```python
from build123d import *

# Parameters (mm, degrees)
SKETCH1_W                 = 108.8
SKETCH1_H                 = 23
MOUNT_BASE_DEPTH          = 5
SKETCH2_R                 = 1
SKETCH2_R_2               = 4.5
BRACKET_SCREW_HOLES_DEPTH = 5
SKETCH3_R                 = 1.5875
ANTENNA_SCREW_HOLES_DEPTH = 5


with BuildPart() as part:
    # Sketch1 → Mount Base (new body)
    with BuildSketch(Plane(origin=(0, 0, 0), x_dir=(1, 0, 0), z_dir=(0, 1, 0))):
        with Locations((54.4, 11.5)):
            Rectangle(SKETCH1_W, SKETCH1_H)
    extrude(amount=MOUNT_BASE_DEPTH)

    # Sketch2 → Bracket Screw Holes (cut)
    with BuildSketch(Plane(origin=(0, 5, 0), x_dir=(1, 0, 0), z_dir=(0, 1, 0))):
        with Locations(Location((59.55, 16.6, 0), (0, 0, 270))):
            Circle(SKETCH2_R)
        with Locations(Location((59.55, 6.4, 0), (0, 0, 270))):
            Circle(SKETCH2_R)
        with Locations(Location((49.25, 6.4, 0), (0, 0, 270))):
            Circle(SKETCH2_R)
        with Locations(Location((49.25, 16.6, 0), (0, 0, 270))):
            Circle(SKETCH2_R)
        with Locations(Location((69.31, 11.5, 0), (0, 0, 270))):
            Circle(SKETCH2_R)
        with Locations(Location((39.49, 11.5, 0), (0, 0, 270))):
            Circle(SKETCH2_R)
        with Locations(Location((54.4, 11.5, 0), (0, 0, 270))):
            Circle(SKETCH2_R_2)
    extrude(amount=-BRACKET_SCREW_HOLES_DEPTH, mode=Mode.SUBTRACT)

    # Sketch3 → Antenna Screw Holes (cut)
    with BuildSketch(Plane(origin=(0, 5, 0), x_dir=(1, 0, 0), z_dir=(0, 1, 0))):
        with Locations(Location((6.7, 11.5, 0), (0, 0, 270))):
            Circle(SKETCH3_R)
        with Locations(Location((24.4, 11.5, 0), (0, 0, 270))):
            Circle(SKETCH3_R)
        with Locations(Location((84.4, 11.5, 0), (0, 0, 270))):
            Circle(SKETCH3_R)
        with Locations(Location((102.1, 11.5, 0), (0, 0, 270))):
            Circle(SKETCH3_R)
    extrude(amount=-ANTENNA_SCREW_HOLES_DEPTH, mode=Mode.SUBTRACT)


solid = part.part
```
Model file for the job. Use its own axes, mm. Coordinates: 2 decimals unless noted, no trailing zeros. Write each loop counter-clockwise with the first axis right and the second up, starting at its lowest first coordinate (ties: lowest second). Pieces come first, ordered by that corner, then holes. Notation, with made-up numbers: (49, 73.25) - (84, 73.25) arc R34 ccw to (84, 111.25) - close; hole circle Ø10 at (26.25, 61). An arc over 180 degrees is marked (long way). One line per question, with ' | ' between items. Start each with the question number.
Q1. Cut at A-A, the plane x = 24.4. List the corners of the cut face in (y, z).
Q2. Pin check, flat tip, straight feed: pin 1 (1.6 mm diameter, centred on x = 49.25, z = -6.4, fed in from +Y). Stop position of the tip, or through.
Q3. Cut at B-B, the plane y = 2.7. Give the number of separate pieces and of enclosed holes in the cut face, then the cut area to 3 significant figures.
Q4. Cut at C-C, the plane x = 54.4. List the corners of the cut face in (y, z), then the cut area to 3 significant figures.
Q5. Drill centre lines: line 1 (X direction, y = 2.2, z = -6.4); line 2 (X direction, y = 2.75, z = -5.75); line 3 (Z direction, x = 52.5, y = 1.4). Where is each one in solid material? Low to high. Write a range as [from, to].
Q6. Pull direction X, two halves, no side cores. Call faces 1 (the face through (53.6, 0, -6.5)), 2 (the face through (108.8, 2, -11)), 3 (the face through (103.674, 2.535, -11.707)): pulls with the +X half, pulls with the -X half, needs draft (parallel to the pull), parting line crosses it, or undercut.
Answer below:
1) outline: (0, -23) - (5, -23) - (5, -13.09) - (0, -13.09) - close; (0, -9.91) - (5, -9.91) - (5, 0) - (0, 0) - close
2) pin 1: through
3) separate pieces: 1 | enclosed holes: 11 | area: 2,390 mm^2
4) outline: (0, -23) - (5, -23) - (5, -16) - (0, -16) - close; (0, -7) - (5, -7) - (5, 0) - (0, 0) - close | area: 70.0 mm^2
5) line 1: [0, 48.25], [50.25, 58.55], [60.55, 108.8] | line 2: [0, 48.49], [50.01, 58.79], [60.31, 108.8] | line 3: [-23, -15.58], [-7.42, 0]
6) face 1: needs draft | face 2: pulls with the +X half | face 3: undercut
